Autodesk Inventor part; units mm, degrees
ref_plane "YZ Plane" through (0, 0, 0) normal (1, 0, 0) x (0, 1, 0)
ref_plane "XZ Plane" through (0, 0, 0) normal (0, 1, 0) x (-1, 0, 0)
ref_plane "XY Plane" through (0, 0, 0) normal (0, 0, 1) x (1, 0, 0)
sketch "Sketch8" plane through (0, 0, 0) normal (0, 0, 1) x (1, 0, 0)
  line L0 (0, 0) -> (0, 15) construction
  line L1 (0, 0) -> (5, 0) construction
  line L2 (5, 0) -> (10, 5) construction
  line L3 (10, 5) -> (20, 5) construction
  line L4 (20, 5) -> (20, 0) construction
  line L5 (21, 0) -> (21, 6)
  line L6 (21, 6) -> (9.5858, 6)
  line L7 (9.5858, 6) -> (4.5858, 1)
  line L8 (4.5858, 1) -> (1, 1)
  line L9 (1, 1) -> (1, 15)
  line L10 (19, 0) -> (19, 4)
  line L11 (19, 4) -> (10.4142, 4)
  line L12 (10.4142, 4) -> (5.4142, -1)
  line L13 (5.4142, -1) -> (-1, -1)
  line L14 (-1, -1) -> (-1, 15)
  line L15 (19, 0) -> (21, 0)
  line L16 (-1, 15) -> (1, 15)
  dimension "d49" = 15
  dimension "d50" = 5
  dimension "d51" = 45
  dimension "d52" = 5
  dimension "d53" = 20
  dimension "d54" = 5
  dimension "d55" = 1
  dimension "d56" = 1
  dimension "d62" = 0
extrude "Extrusion10" add sketch "Sketch8" along normal mid plane 2
sketch "Sketch9" plane through (0, 0, -1) normal (0, 0, -1) x (-1, 0, 0)
  line L0 (1, -1) -> (-5.4142, -1)
  line L1 (-1, 15) -> (1, 15)
  line L2 (-1, 1) -> (-1, 15)
  line L3 (0, 15) -> (0, -1) construction
  circle A0 centre (0, 3.5063) radius 0.75
  dimension "d59" = 1.5
extrude "Extrusion11" add sketch "Sketch9" against normal blind 3.5
sketch "Sketch10" plane through (0, 0, 1) normal (0, 0, 1) x (1, 0, 0)
  line L0 (21, 0) -> (19, 0)
  line L1 (19, 0) -> (19, 4)
  line L2 (5.4142, -1) -> (24, -1) construction
  line L3 (20, 0) -> (20, -1) construction
  line L4 (24, -1) -> (16, -1) construction
  line L5 (16, -1) -> (16, 1)
  line L6 (16, 1) -> (24, 1)
  line L7 (24, 1) -> (24, -1)
  line L8 (20, 0) -> (16.2679, -1)
  line L9 (20, 0) -> (23.7321, -1)
  line L10 (16, -1) -> (16.2679, -1)
  line L11 (23.7321, -1) -> (24, -1)
  dimension "d63" = 2
  dimension "d64" = 4
  dimension "d65" = 8
  dimension "d66" = 15
extrude "Extrusion12" add sketch "Sketch10" against normal up to surface (2 mm away)
sketch "Sketch11" plane through (0, 0, 0) normal (0, 0, 1) x (1, 0, 0)
  line L0 (21, 6) -> (21, 1)
  line L1 (9.5858, 6) -> (21, 6)
  line L2 (4.5858, 1) -> (9.5858, 6)
  line L3 (1, 1) -> (4.5858, 1)
  line L4 (1, 15) -> (1, 1)
  line L5 (-1, 15) -> (1, 15)
  line L6 (-1, -1) -> (-1, 15)
  line L7 (5.4142, -1) -> (-1, -1)
  line L8 (10.4142, 4) -> (5.4142, -1)
  line L9 (19, 4) -> (10.4142, 4)
  line L10 (19, 1) -> (19, 4)
  line L11 (19, 1) -> (16, 1)
  line L12 (16, 1) -> (16, -1)
  line L13 (16, -1) -> (16.2679, -1)
  line L14 (16.2679, -1) -> (20, 0)
  line L15 (20, 0) -> (23.7321, -1)
  line L16 (23.7321, -1) -> (24, -1)
  line L17 (24, -1) -> (24, 1)
  line L18 (24, 1) -> (21, 1)
  line L19 (16, 1) -> (24, 1)
extrude "Extrusion13" add sketch "Sketch11" along normal mid plane 3 contours L18 L17 L16 L15 L14 L13 L12 L11 L19
sketch "Sketch12" plane through (0, 0, -1) normal (0, 0, -1) x (-1, 0, 0)
  circle A0 centre (0, 3.5063) radius 0.75
  circle A1 centre (0, 3.5063) radius 0.75
  circle A2 centre (0, 3.5063) radius 0.5
  dimension "d71" = 1
extrude "Extrusion14" cut sketch "Sketch12" against normal blind 0.1 contours A2
properties part number "SlderC"
Verification items for the finished model (mm, model axes). A direction names the side the tool comes from. Coordinates: 2 decimals unless noted, no trailing zeros. Order: outer loops, then holes, each group sorted by start corner. A loop starts at its lowest first (then second) coordinate and runs counter-clockwise, first axis right, second up. Notation, with made-up numbers: M 31.25,41.25 L 88.25,41.25 A28 cw 88.25,71.25 Z; hole C 31,50.5 d8. An arc over 180 degrees is marked long. One line per item, written item: value. Start each with the question number.
Item 1: Mould release check, pull along X, two halves, no side actions. Record for faces 4 (the flat face through (7.121, 3.535, -0.014)), 5 (the flat face through (15, 6, 0)), 6 (the flat face through (24, 0, 0)): pulls with the +X half, pulls with the -X half, needs draft (parallel to the pull), parting line crosses it, or undercut.
Item 2: Sectioned sample at C-C on x = 0. Record the cut outline in (y, z).
Item 3: Sectioned sample at D-D on x = 18. Record the cut outline in (y, z), then the cut area to 3 significant figures.
Item 4: Sectioned sample at A-A on z = 0.1. Record the cut outline in (x, y), then the cut area to 3 significant figures.
Item 5: Sectioned sample at B-B on y = 5.25. Record the cut outline in (x, z).
Item 6: Depth check by flat-ended pin: P1, Ø8, axis at x = 4.5, y = 3.5, coming from the -Z side; P2, Ø2, axis at x = 21, y = 0, coming from the +Z side; P3, Ø8, axis at x = 9, y = 4, coming from the +Z side. Enter the tip coordinate at first touch or a pass-through.
Item 7: Access from +Z, -Z, +X, -X, +Y, -Y to the whole of each face (thin tool, end or side, straight path). Record for faces 1 (the flat face through (3, 1, 0)), 2 (the flat face through (15, 4, 0)), 3 (the flat face through (21, 3, 0)).
Item 8: Thickness scan on probe 1 along Y at (x, z) = (0, -0.95); probe 2 along Y at (x, z) = (11.75, -0.6); probe 3 along X at (y, z) = (3.5, -0.75). Record the ranges inside material, lowest first.
Calculated:
1. face 4: undercut
1. face 5: needs draft
1. face 6: pulls with the +X half
2. outline: M -1,-1 L 3.01,-1 L 3.01,-0.9 L 4.01,-0.9 L 4.01,-1 L 15,-1 L 15,1 L 4.26,1 L 4.26,2.5 L 2.76,2.5 L 2.76,1 L -1,1 Z
3. outline: M -0.54,-1.5 L 1,-1.5 L 1,1.5 L -0.54,1.5 Z; M 4,-1 L 6,-1 L 6,1 L 4,1 Z
3. area: 8.61 mm^2
4. outline: M -1,-1 L 5.41,-1 L 10.41,4 L 19,4 L 19,1 L 16,1 L 16,-1 L 16.27,-1 L 20,0 L 23.73,-1 L 24,-1 L 24,1 L 21,1 L 21,6 L 9.59,6 L 4.59,1 L 1,1 L 1,15 L -1,15 Z
4. area: 94.4 mm^2
5. outline: M -1,-1 L 1,-1 L 1,1 L -1,1 Z; M 8.84,-1 L 21,-1 L 21,1 L 8.84,1 Z
6. P1: z = -1
6. P2: z = 1.5
6. P3: z = 1
7. face 1: +Z, -Z, +Y
7. face 2: +Z, -Z
7. face 3: +Z, -Z, +X, +Y
8. probe 1: -1 to 3.01, 4.01 to 15
8. probe 2: 4 to 6
8. probe 3: -1 to 1, 7.09 to 9.91, 19 to 21
